from build123d import *

# Parameters (mm, degrees)
BOX_W             = 10
BOX_H             = 10
BOX_DEPTH         = 12
CYLINDER004_R     = 1.5
CYLINDER004_DEPTH = 5
ARRAY_COUNT       = 6
CYLINDER001_R     = 18.5
CYLINDER001_DEPTH = 25
CYLINDER002_R     = 6
CYLINDER002_DEPTH = 6
CYLINDER003_R     = 3
CYLINDER003_DEPTH = 15
CYLINDER_R        = 16
CYLINDER_DEPTH    = 20


with BuildPart() as shaft_d_cut_out:
    # Box → Box (new body)
    with BuildSketch(Plane(origin=(9.5, -5, 9), x_dir=(1, 0, 0), z_dir=(0, 0, 1))):
        with Locations((5, 5)):
            Rectangle(BOX_W, BOX_H)
    extrude(amount=BOX_DEPTH)


with BuildPart() as negative_fusion:
    # Cylinder004 → Cylinder004 (new body)
    with BuildSketch(Plane(origin=(0, -15.5, -5), x_dir=(1, 0, 0), z_dir=(0, 0, 1))):
        Circle(CYLINDER004_R)
    extrude(amount=CYLINDER004_DEPTH)

    # Array: Negative Fusion ×6 about axis
    array_axis = Axis((0, 0, 0), (0, 0, 1))


with BuildPart() as negative_fusion_1:
    add(negative_fusion.part)
    for i in range(1, ARRAY_COUNT):
        add(negative_fusion.part.rotate(array_axis, i * 360 / ARRAY_COUNT))

    # Fusion: union Shaft D Cut Out
    add(shaft_d_cut_out.part)


with BuildPart() as gear_box:
    # Cylinder001 → Cylinder001 (new body)
    with BuildSketch(Plane.XY.offset(-25)):
        Circle(CYLINDER001_R)
    extrude(amount=CYLINDER001_DEPTH)


with BuildPart() as shaft_flange:
    # Cylinder002 → Cylinder002 (new body)
    with BuildSketch(Plane(origin=(7, 0, 0), x_dir=(1, 0, 0), z_dir=(0, 0, 1))):
        Circle(CYLINDER002_R)
    extrude(amount=CYLINDER002_DEPTH)


with BuildPart() as shaft:
    # Cylinder003 → Cylinder003 (new body)
    with BuildSketch(Plane(origin=(7, 0, 6), x_dir=(1, 0, 0), z_dir=(0, 0, 1))):
        Circle(CYLINDER003_R)
    extrude(amount=CYLINDER003_DEPTH)


with BuildPart() as dc_gear_motor_37mm:
    # Cylinder → Cylinder (new body)
    with BuildSketch(Plane.XY.offset(-45)):
        Circle(CYLINDER_R)
    extrude(amount=CYLINDER_DEPTH)

    # Fusion001: union Gear Box, Shaft Flange, Shaft
    add(gear_box.part)
    add(shaft_flange.part)
    add(shaft.part)

    # Cut: cut Negative Fusion
    add(negative_fusion_1.part, mode=Mode.SUBTRACT)


solid = dc_gear_motor_37mm.part
Can you work these out from the model? Positions are in its coordinate system, mm. A direction names the side the tool comes from. Round coordinates to 2 decimals unless told otherwise and drop trailing zeros. Write each loop counter-clockwise with the first axis right and the second up, starting at its lowest first coordinate (ties: lowest second). Pieces come first, ordered by that corner, then holes. Notation, with made-up numbers: M 29.25,39.25 L 76.25,39.25 A7 cw 76.25,51.25 Z; hole C 42.25,-11 d1. An arc over 180 degrees is marked long. Use CSV: the item, a comma, the result in double quotes.
(1) Imagine slicing it at D-D (y = -8). Write out the boundary of the cut face in (x, z).
Check values:
outline,"M -16.68,-25 L -13.86,-25 L -13.86,-45 L 13.86,-45 L 13.86,-25 L 16.68,-25 L 16.68,0 L 14.9,0 L 14.9,-5 L 11.94,-5 L 11.94,0 L -11.94,0 L -11.94,-5 L -14.9,-5 L -14.9,0 L -16.68,0 Z"
(2) Imagine slicing it at A-A (y = 0). Write out the boundary of the cut face in (x, z).
Check values:
outline,"M -18.5,-25 L -16,-25 L -16,-45 L 16,-45 L 16,-25 L 18.5,-25 L 18.5,0 L 13,0 L 13,6 L 10,6 L 10,9 L 9.5,9 L 9.5,21 L 4,21 L 4,6 L 1,6 L 1,0 L -18.5,0 Z"
(3) We'd pull the mould along Y, two halves only. Please class faces 1 (the cylindrical face through (4, 0, 13)), 2 (the cylindrical face through (0, -17, -3)), 3 (the flat face through (7, 0, 21)): +Y half, -Y half, draft (parallel to the pull), parting line (faces both ways), or undercut.
Check values:
face 1,"parting line"
face 2,"undercut"
face 3,"draft"
(4) I need wall thicknesses on line 1 along Y through (x, z) = (0, -0.95); line 2 along X through (y, z) = (7, -1); line 3 along Z through (x, y) = (-2.5, 13). Which ranges of each line are inside material? Lowest first, please.
Check values:
line 1,"-18.5 to -17, -14 to 14, 17 to 18.5"
line 2,"-17.12 to -14.72, -12.12 to 12.12, 14.72 to 17.12"
line 3,"-45 to 0"
(5) I'm going to push flat-ended pins straight in: pin 1 (0.9 mm diameter, centred on x = -0.5, y = 15.5, fed in from +Z); pin 2 (3.5 mm diameter, centred on x = 13, y = -7.5, fed in from +Z); pin 3 (12 mm diameter, centred on y = 12, z = -36, fed in from -X). Where does each tip first touch, or does it pass through?
Check values:
pin 1,"z = -5"
pin 2,"z = 0"
pin 3,"x = -14.83"
(6) Imagine slicing it at B-B (x = 0). Write out the boundary of the cut face in (y, z), plus the area to 4 significant figures.
Check values:
outline,"M -18.5,-25 L -16,-25 L -16,-45 L 16,-45 L 16,-25 L 18.5,-25 L 18.5,0 L 17,0 L 17,-5 L 14,-5 L 14,0 L -14,0 L -14,-5 L -17,-5 L -17,0 L -18.5,0 Z"
area,"1,535 mm^2"
(7) Imagine slicing it at C-C (z = -3.5). Write out the boundary of the cut face in (x, y).
Check values:
outline,"C 0,0 d37; hole C -13.42,-7.75 d3; hole C -13.42,7.75 d3; hole C 0,-15.5 d3; hole C 0,15.5 d3; hole C 13.42,-7.75 d3; hole C 13.42,7.75 d3"
(8) On a 3-axis mill with a long thin cutter (end or side, diameter ignored), from which of +Z, -Z, +X, -X, +Y, -Y can I reach the whole of each face in a straight line? I mean faces 4 (the flat face through (9.5, 0, 15)), 5 (the flat face through (0, 0, -45)), 6 (the cylindrical face through (-4.01, -18.06, -12.68)), 7 (the cylindrical face through (12.617, -9.015, -2.535)), 8 (the cylindrical face through (-3.47, -15.62, -35.14)). Say none if no direction works.
Check values:
face 4,"+Z, +X, +Y, -Y"
face 5,"-Z, +X, -X, +Y, -Y"
face 6,"+Z, -Z"
face 7,"+Z"
face 8,"-Z"
